Check sheet for the modelled part. Datum: model origin and axes. Units: mm. Face numbers are marked on the shaded views. A direction names the side the tool comes from. Round coordinates to 2 decimals unless told otherwise and drop trailing zeros. Write each loop counter-clockwise with the first axis right and the second up, starting at its lowest first coordinate (ties: lowest second). Pieces come first, ordered by that corner, then holes.
Item 1: Release check for a two-part mould opening along X. For the marked faces 3, 4 and 5 record: pulls with the +X half, pulls with the -X half, needs draft (parallel to the pull), parting line crosses it, or undercut.
Item 2: Set-up check for the marked faces 1 and 2: record each of +Z, -Z, +X, -X, +Y, -Y from which the full face is reachable in a straight line by a thin tool's end or side.
Item 3: Section check D-D, the plane x = 43. Record the cut outline in (y, z), plus the area to 3 significant figures.
Item 4: Material ranges on line 1 along X through (y, z) = (22.5, 5.75); line 2 along X through (y, z) = (-29, -2.25); line 3 along X through (y, z) = (45, 3.5), recorded low to high.
Item 5: Depth check by flat-ended pin: pin 1 (6 mm diameter, centred on x = 33.5, z = 6.5, fed in from -Y); pin 2 (4 mm diameter, centred on y = -30, z = -3, fed in from +X); pin 3 (1 mm diameter, centred on y = 18, z = -3.5, fed in from -X); pin 4 (18 mm diameter, centred on x = 39.95, y = 39.95, fed in from -Z). Enter the tip coordinate at first touch or a pass-through.
Item 6: Section check C-C, the plane y = -7. Record the cut outline in (x, z).
Item 7: Section check B-B, the plane x = -3. Record the cut outline in (y, z).
from build123d import *

# Parameters (mm, degrees)
BOSS_EXTRUDE1_DEPTH = 10


with BuildPart() as part:
    # Sketch1 → Boss-Extrude1 (new, symmetric)
    with BuildSketch(Plane.XY):
        with BuildLine():
            ThreePointArc((5.499886369, 31.523820357), (0, 32), (-5.499886369, 31.523820357))
            ThreePointArc((-5.499886369, 31.523820357), (-18.956279365, 33.916662735), (-27.733810979, 44.393071751))
            ThreePointArc((-27.733810979, 44.393071751), (-49.143921292, 49.143921292), (-44.393071751, 27.733810979))
            ThreePointArc((-44.393071751, 27.733810979), (-33.916662735, 18.956279365), (-31.523820357, 5.499886369))
            ThreePointArc((-31.523820357, 5.499886369), (-32, 0), (-31.523820357, -5.499886369))
            ThreePointArc((-31.523820357, -5.499886369), (-33.916662735, -18.956279365), (-44.393071751, -27.733810979))
            ThreePointArc((-44.393071751, -27.733810979), (-49.143921292, -49.143921292), (-27.733810979, -44.393071751))
            ThreePointArc((-27.733810979, -44.393071751), (-18.956279365, -33.916662735), (-5.499886369, -31.523820357))
            ThreePointArc((-5.499886369, -31.523820357), (0, -32), (5.499886369, -31.523820357))
            ThreePointArc((5.499886369, -31.523820357), (18.956279365, -33.916662735), (27.733810979, -44.393071751))
            ThreePointArc((27.733810979, -44.393071751), (49.143921292, -49.143921292), (44.393071751, -27.733810979))
            ThreePointArc((44.393071751, -27.733810979), (33.916662735, -18.956279365), (31.523820357, -5.499886369))
            ThreePointArc((31.523820357, -5.499886369), (32, 0), (31.523820357, 5.499886369))
            ThreePointArc((31.523820357, 5.499886369), (33.916662735, 18.956279365), (44.393071751, 27.733810979))
            ThreePointArc((44.393071751, 27.733810979), (49.143921292, 49.143921292), (27.733810979, 44.393071751))
            ThreePointArc((27.733810979, 44.393071751), (18.956279365, 33.916662735), (5.499886369, 31.523820357))
        make_face()
        with BuildLine():
            Line((37.363342686, 30.292274874), (22.297196945, 15.226129133))
            ThreePointArc((22.297196945, 15.226129133), (27, 0), (22.297196945, -15.226129133))
            Line((22.297196945, -15.226129133), (37.363342686, -30.292274874))
            ThreePointArc((37.363342686, -30.292274874), (47.022600949, -47.022600949), (30.292274874, -37.363342686))
            Line((30.292274874, -37.363342686), (15.226129133, -22.297196945))
            ThreePointArc((15.226129133, -22.297196945), (0, -27), (-15.226129133, -22.297196945))
            Line((-15.226129133, -22.297196945), (-30.292274874, -37.363342686))
            ThreePointArc((-30.292274874, -37.363342686), (-47.022600949, -47.022600949), (-37.363342686, -30.292274874))
            Line((-37.363342686, -30.292274874), (-22.297196945, -15.226129133))
            ThreePointArc((-22.297196945, -15.226129133), (-27, 0), (-22.297196945, 15.226129133))
            Line((-22.297196945, 15.226129133), (-37.363342686, 30.292274874))
            ThreePointArc((-37.363342686, 30.292274874), (-47.022600949, 47.022600949), (-30.292274874, 37.363342686))
            Line((-30.292274874, 37.363342686), (-15.226129133, 22.297196945))
            ThreePointArc((-15.226129133, 22.297196945), (0, 27), (15.226129133, 22.297196945))
            Line((15.226129133, 22.297196945), (30.292274874, 37.363342686))
            ThreePointArc((30.292274874, 37.363342686), (47.022600949, 47.022600949), (37.363342686, 30.292274874))
        make_face(mode=Mode.SUBTRACT)
    extrude(amount=BOSS_EXTRUDE1_DEPTH, both=True)


solid = part.part
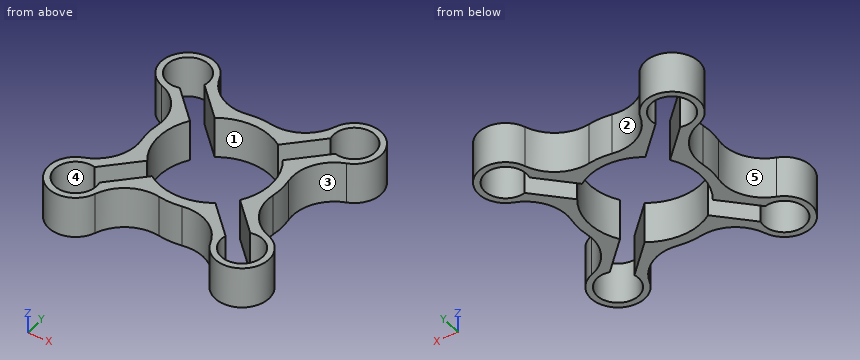
Values found:
1. face 3: pulls with the +X half
1. face 4: undercut
1. face 5: pulls with the -X half
2. face 1: +Z, -Z
2. face 2: +Z, -Z, +Y
3. outline: (-52.59, -10) - (-49.48, -10) - (-49.48, 10) - (-52.59, 10) - close; (-30.43, -10) - (-27.17, -10) - (-27.17, 10) - (-30.43, 10) - close; (27.17, -10) - (30.43, -10) - (30.43, 10) - (27.17, 10) - close; (49.48, -10) - (52.59, -10) - (52.59, 10) - (49.48, 10) - close
3. area: 255 mm2
4. line 1: x = -36.53 to -29.57, -15.43 to -14.92, 14.92 to 15.43, 29.57 to 36.53
4. line 2: x = -46.96 to -36.07, -21.93 to 21.93, 36.07 to 46.96
4. line 3: x = -51.93 to -48.58, -31.32 to -27.97, 27.97 to 31.32, 48.58 to 51.93
5. pin 1: stops at y = -52.48
5. pin 2: stops at x = 50.24
5. pin 3: stops at x = -33.66
5. pin 4: passes through
6. outline: (-31.32, -10) - (-26.08, -10) - (-26.08, 10) - (-31.32, 10) - close; (26.08, -10) - (31.32, -10) - (31.32, 10) - (26.08, 10) - close
7. outline: (-31.86, -10) - (-26.83, -10) - (-26.83, 10) - (-31.86, 10) - close; (26.83, -10) - (31.86, -10) - (31.86, 10) - (26.83, 10) - close
